Here's how the part is built. I have some questions about the finished solid (model axes, mm). A direction names the side the tool comes from. Give positions to 0.01 mm unless a question says otherwise; leave off trailing zeros. Order: outer loops, then holes, each group sorted by start corner. A loop starts at its lowest first (then second) coordinate and runs counter-clockwise, first axis right, second up. Notation, with made-up numbers: (-28.5, 8) - (-15.5, 8) arc R18 cw to (-15.5, 25) - close; hole circle Ø10 at (-1.75, 40). An arc over 180 degrees is marked (long way). One line per question, with ' | ' between items.
from build123d import *

# Parameters (mm, degrees)
CROQUIS1_W              = 33
CROQUIS1_H              = 58
CROQUIS1_W_2            = 25
CROQUIS1_H_2            = 50
SALIENTE_EXTRUIR1_DEPTH = 70
CROQUIS2_W              = 33
CROQUIS2_H              = 58
SALIENTE_EXTRUIR2_DEPTH = 3
CROQUIS3_W              = 33
CROQUIS3_H              = 4
CORTAR_EXTRUIR1_DEPTH   = 81.263628126


with BuildPart() as part:
    # Croquis1 → Saliente-Extruir1 (new body)
    with BuildSketch(Plane.XY):
        Rectangle(CROQUIS1_W, CROQUIS1_H)
        Rectangle(CROQUIS1_W_2, CROQUIS1_H_2, mode=Mode.SUBTRACT)
    extrude(amount=SALIENTE_EXTRUIR1_DEPTH)

    # Croquis2 → Saliente-Extruir2 (add)
    with BuildSketch(Plane(origin=(0, 0, 0), x_dir=(-1, 0, 0), z_dir=(0, 0, -1))):
        Rectangle(CROQUIS2_W, CROQUIS2_H)
    extrude(amount=SALIENTE_EXTRUIR2_DEPTH)

    # Croquis3 → Cortar-Extruir1 (cut, through all)
    with BuildSketch(Plane.XY.offset(70)):
        with Locations((0, -27)):
            Rectangle(CROQUIS3_W, CROQUIS3_H)
    extrude(amount=-CORTAR_EXTRUIR1_DEPTH, mode=Mode.SUBTRACT)


solid = part.part
1) Thinking about a two-plate mould opening in X: for faces 1 (the face through (-14, 8, 70)), 2 (the face through (0, 25, 35)), 3 (the face through (-16.5, 2, 34)), which applies, +X half, -X half, draft (parallel to the pull), parting line (faces both ways), or undercut?
Model answer:
face 1: draft | face 2: undercut | face 3: -X half
2) I want a section at B-B (x = 1). List the corners of the cut face in (y, z) for me.
Model answer:
outline: (-25, -3) - (29, -3) - (29, 70) - (25, 70) - (25, 0) - (-25, 0) - close
3) I want a section at C-C (y = 11). List the corners of the cut face in (x, z) for me.
Model answer:
outline: (-16.5, -3) - (16.5, -3) - (16.5, 70) - (12.5, 70) - (12.5, 0) - (-12.5, 0) - (-12.5, 70) - (-16.5, 70) - close
4) I want a section at A-A (z = 39). List the corners of the cut face in (x, y) for me.
Model answer:
outline: (-16.5, -25) - (-12.5, -25) - (-12.5, 25) - (12.5, 25) - (12.5, -25) - (16.5, -25) - (16.5, 29) - (-16.5, 29) - close
5) On a 3-axis mill with a long thin cutter (end or side, diameter ignored), from which of +Z, -Z, +X, -X, +Y, -Y can I reach the whole of each face in a straight line? I mean faces 4 (the face through (0, 2, -3)), 5 (the face through (12.5, 0, 35)). Say none if no direction works.
Model answer:
face 4: -Z, +X, -X, +Y, -Y | face 5: +Z, -Y
6) Please list where these lines run through material, in increasing order: L1, parallel to X at y = 16, z = 60.5; L2, parallel to Y at x = 8.5, z = 45; L3, parallel to Z at x = 2, y = -19.5.
Model answer:
L1: x = -16.5 to -12.5, 12.5 to 16.5 | L2: y = 25 to 29 | L3: z = -3 to 0
7) I'm going to push flat-ended pins straight in: P1, Ø7.5, axis at x = -4.5, z = 42.5, coming from the -Y side; P2, Ø12, axis at x = 0, y = -4, coming from the +Z side. Where does each tip first touch, or does it pass through?
Model answer:
P1: stops at y = 25 | P2: stops at z = 0
